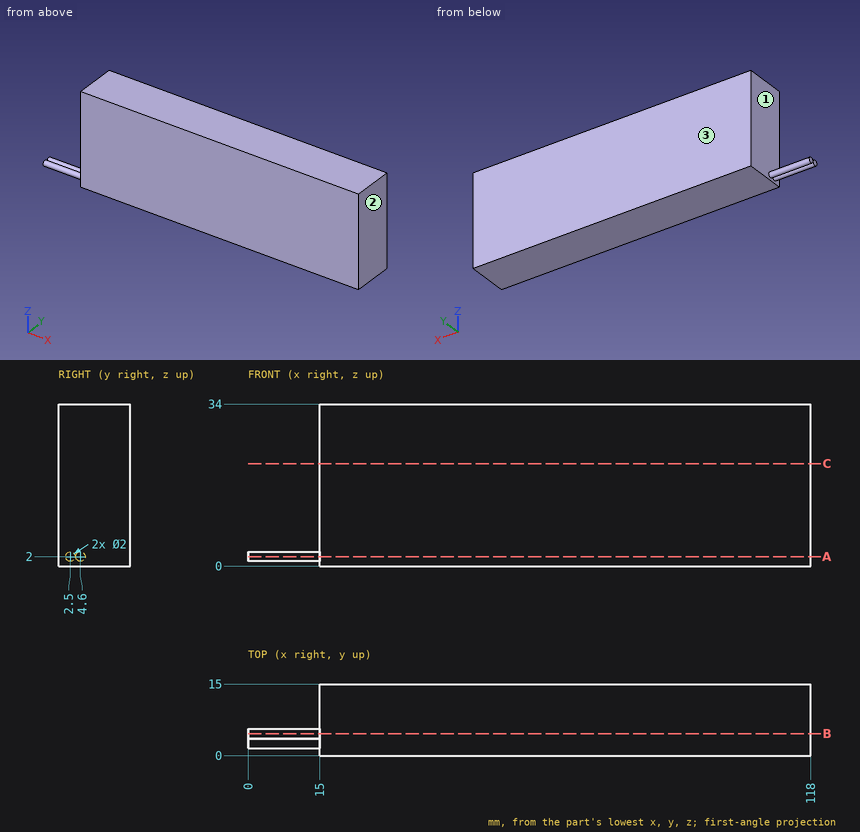
Part print with two shaded views. Sizes in mm from the minimum x, y, z corner. Coordinates: 2 decimals unless noted, no trailing zeros. Write each loop counter-clockwise with the first axis right and the second up, starting at its lowest first coordinate (ties: lowest second). Pieces come first, ordered by that corner, then holes. Notation, with made-up numbers: M 71.5,79.25 L 106.5,79.25 A24 ccw 106.5,89.25 Z; hole C 11.25,15 d4. An arc over 180 degrees is marked long. Return JSON: item names as keys, results as strings.
Item 1: Slice it at B-B, the plane y = 4.6. Write the cut outline in (x, z).
Findings below:
{"outline": "M 0,1 L 15,1 L 15,0 L 118,0 L 118,34 L 15,34 L 15,3 L 0,3 Z"}
Item 2: Drop flat-ended pins along their axis: pin 1 Ø6 at (y, z) = (2, 8) entering from -X; pin 2 Ø5 at (x, y) = (47, 7) entering from -Z. Give the stop position or say it passes through.
Findings below:
{"pin 1": "stops at x = 15", "pin 2": "stops at z = 0"}
Item 3: Two-plate mould, pull along X, no slides. Class the marked faces 1, 2 and 3: +X half, -X half, draft (parallel to the pull), parting line (faces both ways), or undercut.
Findings below:
{"face 1": "-X half", "face 2": "+X half", "face 3": "draft"}
Item 4: Slice it at C-C, the plane z = 21.5. Write the cut outline in (x, y).
Findings below:
{"outline": "M 15,0 L 118,0 L 118,15 L 15,15 Z"}
Item 5: Slice it at A-A, the plane z = 2. Write the cut outline in (x, y), and give its area (4 significant figures).
Findings below:
{"outline": "M 0,1.5 L 15,1.5 L 15,0 L 118,0 L 118,15 L 15,15 L 15,5.6 L 0,5.6 L 0,3.6 L 15,3.6 L 15,3.5 L 0,3.5 Z", "area": "1,605 mm2"}
Item 6: Probe line 1 (X direction, y = 14.25, z = 24); line 2 (Z direction, x = 8.5, y = 3). List the from-to ranges inside material, lowest first. Write a range as from..to.
Findings below:
{"line 1": "x = 15..118", "line 2": "z = 1.13..2.87"}
